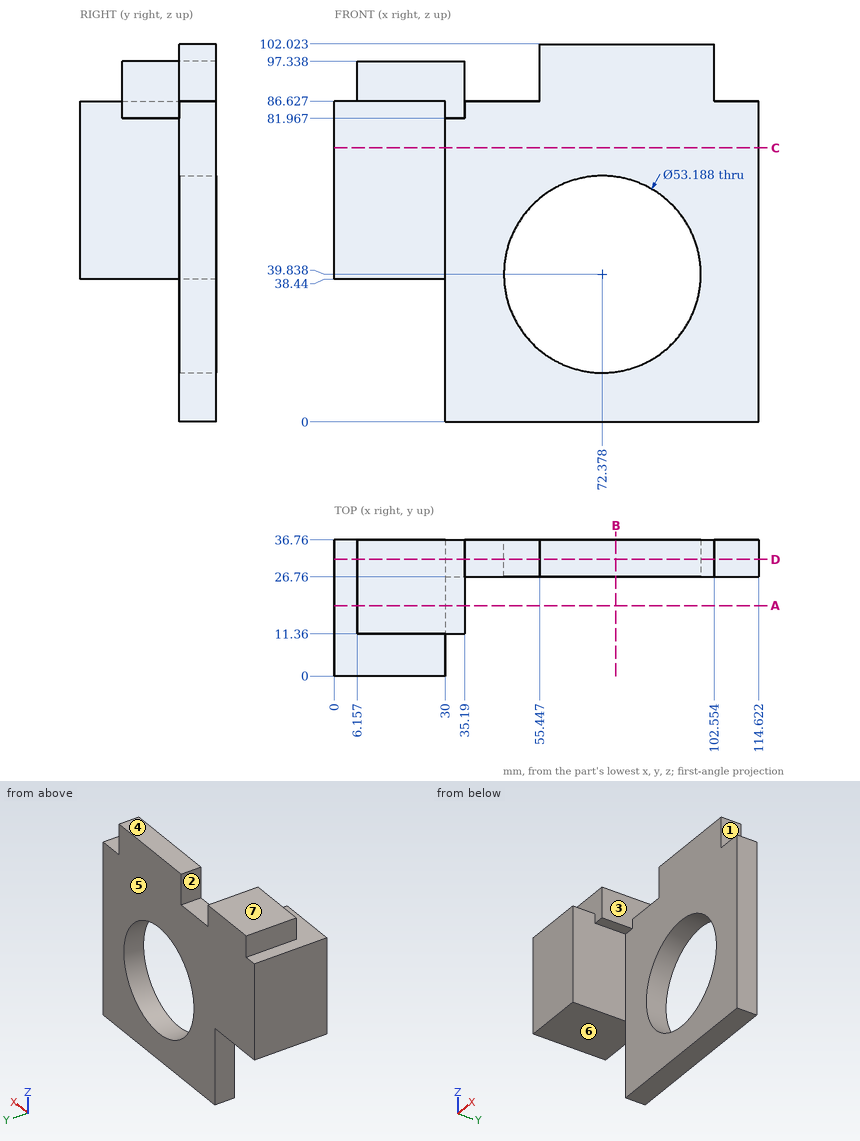
Geometry check sheet. Reference: drawing and pictorial views, mm from the part's lowest x, y, z. A direction names the side the tool comes from. Round coordinates to 2 decimals unless told otherwise and drop trailing zeros. Loops run counter-clockwise (first coordinate to the right, second up) from the corner with the lowest first, then second, coordinate; pieces in that order, holes last. Notation, with made-up numbers: M 21,-6.75 L 62,-6.75 A21 ccw 62,14.25 Z; hole C 55,-22.75 d3. An arc over 180 degrees is marked long. Return JSON: item names as keys, results as strings. Group by question number.
(1) Section check C-C, the plane z = 74. Enter the section's corners in (x, y), and give its area (3 significant figures).
(2) Section check D-D, the plane y = 31.5. Enter the section's corners in (x, z).
(3) Mould release check, pull along X, two halves, no side actions. Record for the marked faces 1, 2, 3 and 4: pulls with the +X half, pulls with the -X half, needs draft (parallel to the pull), parting line crosses it, or undercut.
(4) Scan lines: line 1 along X through (y, z) = (33.5, 89.5); line 2 along X through (y, z) = (9, 78); line 3 along Z through (x, y) = (11, 28). Record each from-to range of solid material in increasing order. Write a range as [from, to].
(5) Go/stop test with flat-tipped pins: pin 1 (1.5 mm diameter, centred on y = 28, z = 35, fed in from -X); pin 2 (5 mm diameter, centred on x = 107.5, y = 34, fed in from +Z); pin 3 (5 mm diameter, centred on x = 49, z = 28, fed in from -Y). Record where each tip stops, or that it passes through.
(6) Set-up check for the marked faces 5, 6 and 7: record each of +Z, -Z, +X, -X, +Y, -Y from which the full face is reachable in a straight line by a thin tool's end or side.
(7) Section check B-B, the plane x = 76. Enter the section's corners in (y, z).
(8) Section check A-A, the plane y = 19. Enter the section's corners in (x, z).
Data:
{
 "1": {"outline": "M 0,0 L 30,0 L 30,26.76 L 114.62,26.76 L 114.62,36.76 L 0,36.76 Z", "area": "1,950 mm²"},
 "2": {"outline": "M 0,38.44 L 30,38.44 L 30,0 L 114.62,0 L 114.62,86.63 L 102.55,86.63 L 102.55,102.02 L 55.45,102.02 L 55.45,86.63 L 35.19,86.63 L 35.19,97.34 L 6.16,97.34 L 6.16,86.63 L 0,86.63 Z; hole C 72.38,39.84 d53.19"},
 "3": {"face 1": "pulls with the +X half", "face 2": "undercut", "face 3": "undercut", "face 4": "needs draft"},
 "4": {"line 1": "[6.16, 35.19], [55.45, 102.55]", "line 2": "[0, 30]", "line 3": "[38.44, 97.34]"},
 "5": {"pin 1": "x = 30", "pin 2": "z = 86.63", "pin 3": "y = 26.76"},
 "6": {"face 5": "+Z, -Z, +X, -X, +Y", "face 6": "-Z, -X, +Y, -Y", "face 7": "+Z, -X, +Y, -Y"},
 "7": {"outline": "M 26.76,0 L 36.76,0 L 36.76,13.49 L 26.76,13.49 Z; M 26.76,66.18 L 36.76,66.18 L 36.76,102.02 L 26.76,102.02 Z"},
 "8": {"outline": "M 0,38.44 L 30,38.44 L 30,81.97 L 35.19,81.97 L 35.19,97.34 L 6.16,97.34 L 6.16,86.63 L 0,86.63 Z"}
}
